Work out the finished part from the listing and answer in its coordinate system (mm). Give positions to 0.01 mm unless a question says otherwise; leave off trailing zeros. Order: outer loops, then holes, each group sorted by start corner. A loop starts at its lowest first (then second) coordinate and runs counter-clockwise, first axis right, second up.
```python
from build123d import *

# Parameters (mm, degrees)
F0_R     = 10
F0_R_2   = 5
F1_DEPTH = 4
F2_R     = 10
F2_R_2   = 9
F3_DEPTH = 12
F5_R     = 10
F6_DEPTH = 1
F7_R     = 2
F8_DEPTH = 10


# Not quite as in the source:
# - a fillet or chamfer that OpenCascade refuses, or shapes differently, is made with other operations: its cross-section is extruded or revolved along the edge and cut away or added


with BuildPart() as f1:
    # F0 (on Top) → F1 (new body)
    with BuildSketch(Plane.XY):
        Circle(F0_R)
        Circle(F0_R_2, mode=Mode.SUBTRACT)
    extrude(amount=F1_DEPTH)

    # F2 (on Top) → F3 (join)
    with BuildSketch(Plane.XY):
        Circle(F2_R)
        Circle(F2_R_2, mode=Mode.SUBTRACT)
    extrude(amount=F3_DEPTH)

    # F4: fillet of radius 5 on 1 edges, made by hand

    # F4_s1 → F4_t2 (revolve, cut)
    with BuildSketch(Plane.XZ):
        with BuildLine():
            ThreePointArc((10, 9), (9.7434164903, 10.5811388301), (9, 12))
            Line((9, 12), (10, 12))
            Line((10, 12), (10, 9))
        make_face()
    revolve(axis=Axis((0, 0, 12), (0, 0, 1)), mode=Mode.SUBTRACT)

    # F5 (on face) → F6 (join)
    with BuildSketch(Plane.XY):
        Circle(F5_R)
    extrude(amount=-F6_DEPTH)

    # F7
    f7_edges = [f1.edges().sort_by_distance(p)[0] for p in [
        (-10, 0, -1),
    ]]
    fillet(f7_edges, radius=F7_R)

    # F0 (on Top) → F8 (join)
    with BuildSketch(Plane.XY):
        Circle(F0_R_2)
        with BuildLine():
            ThreePointArc((1.65, -2.683281573), (-3.15, 0), (1.65, 2.683281573))
            Line((1.65, 2.683281573), (1.65, -2.683281573))
        make_face(mode=Mode.SUBTRACT)
    extrude(amount=F8_DEPTH)


solid = f1.part
```
1. The mould has two halves that part along X. Classify faces 1 (the face through (5.38, 8.43, 4.94)), 2 (the face through (-1.08, -4.88, 6.96)), 3 (the face through (0, 0, -1)): pulls with the +X half, pulls with the -X half, needs draft (parallel to the pull), parting line crosses it, or undercut.
Findings below:
face 1: parting line crosses it
face 2: undercut
face 3: needs draft
2. Given P1, Ø3, axis at y = 0.5, z = 10, coming from the +X side; P2, Ø3, axis at x = -0.5, y = 0, coming from the +Z side; P3, Ø5.5, axis at x = -0.5, y = 1, coming from the +Z side; P4, Ø2, axis at x = 3.5, z = 8, coming from the +Y side, each flat-ended and moving along its own axis, determine where each tip first touches the part or whether it passes through.
Findings below:
P1: stops at x = 10
P2: stops at z = 0
P3: stops at z = 10
P4: stops at y = 9.68
3. The part is cut by section B-B (z = 3.25). Write down the section's boundary in (x, y), then the cut area to 3 significant figures.
Findings below:
outline: circle Ø20 at (0, 0); hole (1.65, -2.68) - (1.65, 2.68) arc R3.15 ccw (long way) to start
area: 289 mm2
4. The part is cut by section A-A (z = 4.75). Write down the section's boundary in (x, y).
Findings below:
outline: circle Ø20 at (0, 0); circle Ø10 at (0, 0); hole circle Ø18 at (0, 0); hole (1.65, -2.68) - (1.65, 2.68) arc R3.15 ccw (long way) to start
5. The part is cut by section C-C (z = 10.75). Write down the section's boundary in (x, y), then the cut area to 3 significant figures.
Findings below:
outline: circle Ø19.37 at (0, 0); hole circle Ø18 at (0, 0)
area: 40.1 mm2
6. Straight lines are drawn through the part: probe 1 along Y at (x, z) = (0, 8.5); probe 2 along X at (y, z) = (-0.75, 7); probe 3 along Y at (x, z) = (-4, 6.5). For each, find the intervals that lie inside material, in ascending order.
Findings below:
probe 1: y = -10 to -9, -5 to -3.15, 3.15 to 5, 9 to 10
probe 2: x = -9.97 to -8.97, -4.94 to -3.06, 1.65 to 4.94, 8.97 to 9.97
probe 3: y = -9.17 to -8.06, -3 to 3, 8.06 to 9.17
